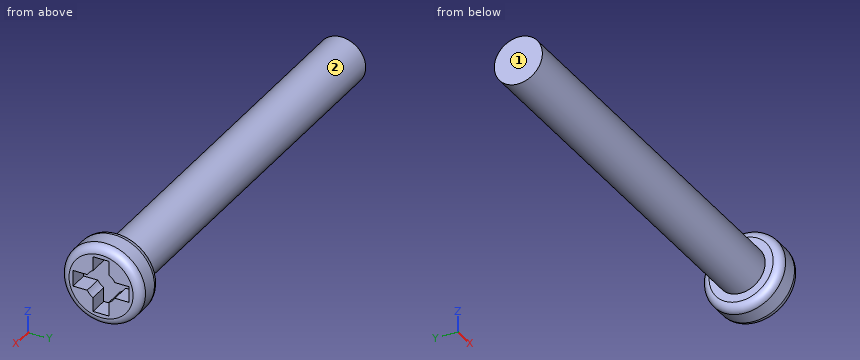
Autodesk Inventor part; units mm, degrees
ref_plane "YZ Plane" through (0, 0, 0) normal (1, 0, 0) x (0, 1, 0)
ref_plane "XZ Plane" through (0, 0, 0) normal (0, 1, 0) x (-1, 0, 0)
ref_plane "XY Plane" through (0, 0, 0) normal (0, 0, 1) x (1, 0, 0)
sketch "Sketch1" plane through (0, 0, 0) normal (1, 0, 0) x (0, 1, 0)
  circle A0 centre (0, 0) radius 1.5
  dimension "d0" = 3
extrude "Extrusion1" add sketch "Sketch1" against normal blind 25
sketch "Sketch2" plane through (0, 0, 0) normal (1, 0, 0) x (0, 0, -1)
  circle A0 centre (0, 0) radius 2.5
  dimension "d3" = 5
extrude "Extrusion2" add sketch "Sketch2" along normal blind 2
fillet "Fillet1" radius 0.5 2 edges at (0, 0, 2.5) (2, 0, 2.5)
sketch "Sketch3" plane through (2, 0, 0) normal (1, 0, 0) x (0, 0, -1)
  line L0 (1.75, -0.5) -> (1.75, 0.5)
  line L1 (-1.75, 0.5) -> (-1.75, -0.5)
  line L2 (0.5, 1.75) -> (-0.5, 1.75)
  line L3 (-0.5, -1.75) -> (0.5, -1.75)
  line L4 (-0.5, 1.75) -> (-0.5, 0.866)
  line L5 (-0.5, -0.866) -> (-0.5, -1.75)
  line L6 (-1.75, -0.5) -> (-0.866, -0.5)
  line L7 (0.866, -0.5) -> (1.75, -0.5)
  line L8 (1.75, 0.5) -> (0.866, 0.5)
  line L9 (-0.866, 0.5) -> (-1.75, 0.5)
  line L10 (0.5, -1.75) -> (0.5, -0.866)
  line L11 (0.5, 0.866) -> (0.5, 1.75)
  arc A0 (-0.5, 0.866) -> (-0.866, 0.5) centre (0, 0) ccw
  arc A1 (-0.866, -0.5) -> (-0.5, -0.866) centre (0, 0) ccw
  arc A2 (0.5, -0.866) -> (0.866, -0.5) centre (0, 0) ccw
  arc A3 (0.866, 0.5) -> (0.5, 0.866) centre (0, 0) ccw
  dimension "d7" = 3.5
  dimension "d8" = 1
  dimension "d9" = 3.5
  dimension "d10" = 1
extrude "Extrusion3" cut sketch "Sketch3" against normal blind 1.2
thread "Thread1"
properties part number "Parafuso lateral do captador"
Input: part model. Units: mm. Frame: model coordinates. Face numbers are marked on the shaded views. A direction names the side the tool comes from. Coordinates: 2 decimals unless noted, no trailing zeros. Loops run counter-clockwise (first coordinate to the right, second up) from the corner with the lowest first, then second, coordinate; pieces in that order, holes last. Notation, with made-up numbers: (59.5, 78) -> (68.5, 78) arc R19 cw to (68.5, 106) -> close; hole circle Ø11 at (39.5, 50). An arc over 180 degrees is marked (long way). Write item = value, one per line. Start each with the question number.
Item 1: Cut plane A-A, the plane z = 0. Return loops of the section in (x, y), plus the area to 3 significant figures.
Item 2: Reachability of the marked faces 1 and 2 from +Z, -Z, +X, -X, +Y, -Y: full face, straight path, thin tool, end or side. Return the list, or none.
Item 3: Material intervals for line 1 (X direction, y = 0.3, z = 0.5); line 2 (X direction, y = 1.5, z = -0.8); line 3 (Z direction, x = -13, y = 0), sorted ascending.
Item 4: First-contact query: P1, Ø1.5, axis at x = -20.5, z = 2, coming from the +Y side; P2, Ø1, axis at x = 1.5, z = 1.5, coming from the -Y side; P3, Ø3, axis at x = -11, y = -1.5, coming from the -Z side; P4, Ø1.8, axis at y = 0, z = -0.5, coming from the +X side. Flat tips, straight axial feed; report the tip coordinate or a pass-through.
Item 5: Cut plane C-C, the plane x = -10. Return loops of the section in (y, z), plus the area to 3 significant figures.
Ans:
q1.outline = (-25, -1.5) -> (0, -1.5) -> (0, -2) arc R0.5 ccw to (0.5, -2.5) -> (1.5, -2.5) arc R0.5 ccw to (2, -2) -> (2, -1.75) -> (0.8, -1.75) -> (0.8, 1.75) -> (2, 1.75) -> (2, 2) arc R0.5 ccw to (1.5, 2.5) -> (0.5, 2.5) arc R0.5 ccw to (0, 2) -> (0, 1.5) -> (-25, 1.5) -> close
q1.area = 80.6 mm²
q2.face_1 = +Z, -Z, -X, +Y, -Y
q2.face_2 = -X
q3.line_1 = -25 to 0.8
q3.line_2 = 0 to 2
q3.line_3 = -1.5 to 1.5
q4.P1 = 0.83
q4.P2 = -2.29
q4.P3 = -1.5
q4.P4 = 2
q5.outline = circle Ø3 at (0, 0)
q5.area = 7.07 mm²
